Model file for the job. Use its own axes, mm. A direction names the side the tool comes from. Coordinates: 2 decimals unless noted, no trailing zeros. Order: outer loops, then holes, each group sorted by start corner. A loop starts at its lowest first (then second) coordinate and runs counter-clockwise, first axis right, second up. Notation, with made-up numbers: (30.25, 40) -> (64.25, 40) arc R16 ccw to (64.25, 67) -> close; hole circle Ø9 at (-9, 48.25). An arc over 180 degrees is marked (long way). Return JSON: item names as keys, results as strings. Group by question number.
1) Flat gauge pin, fed straight in: pin 1 (10 mm diameter, centred on x = 116.3, y = 53.8, fed in from -Z). Where does the tip first touch, or does it go through?
2) Probe line 1 (Y direction, x = 0, z = 2.1) (3 decimals); line 2 (Y direction, x = 94, z = 0.4); line 3 (X direction, y = 12, z = 2.95). List the from-to ranges inside material, lowest first.
3) Pull direction X, two halves, no side cores. Call faces 1 (the cylindrical face through (123.09, -60.69, 1.57)), 2 (the flat face through (-2, 43, 0)), 3 (the cylindrical face through (55.63, -55.73, 1.57)): +X half, -X half, draft (parallel to the pull), parting line (faces both ways), or undercut.
4) Cut at A-A (x = 15). Write the cut outline in (y, z) (3 decimals), and give its area (3 significant figures).
5) Which spindle directions (+Z, -Z, +X, -X, +Y, -Y) get a long thin tool onto all of the face, cutting with end or side? Do faces 4 (the flat face through (-2, 43, 3.175)), 5 (the cylindrical face through (-97.69, -35.29, 1.57)). Say none if no direction does.
6) Cut at C-C (z = 2.2). State how many separate pieces and enclosed holes the cut face has, and give its area (3 significant figures).
7) Cut at B-B (y = -9.5). Write the cut outline in (x, z) (3 decimals), and give its area (3 significant figures).
from build123d import *

# Parameters (mm, degrees)
F0_R     = 3.175
F1_DEPTH = 3.175


with BuildPart() as f1:
    # F0 (on Top) → F1 (new body)
    with BuildSketch(Plane.XY):
        with BuildLine():
            Line((118.650004, 62.500002), (-118.650004, 62.500002))
            ThreePointArc((-118.650004, 62.500002), (-123.140132, 60.64013), (-125.000004, 56.150002))
            Line((-125.000004, 56.150002), (-125.000004, -56.150002))
            ThreePointArc((-125.000004, -56.150002), (-123.140132, -60.64013), (-118.650004, -62.500002))
            Line((-118.650004, -62.500002), (118.650004, -62.500002))
            ThreePointArc((118.650004, -62.500002), (123.140132, -60.64013), (125.000004, -56.150002))
            Line((125.000004, -56.150002), (125.000004, 56.150002))
            ThreePointArc((125.000004, 56.150002), (123.140132, 60.64013), (118.650004, 62.500002))
        make_face()
        with Locations((-116.299996, -53.79999)):
            Circle(F0_R, mode=Mode.SUBTRACT)
        with Locations((-58.149998, -53.79999)):
            Circle(F0_R, mode=Mode.SUBTRACT)
        with Locations((-116.299996, -4e-06)):
            Circle(F0_R, mode=Mode.SUBTRACT)
        with Locations((0, -53.79999)):
            Circle(F0_R, mode=Mode.SUBTRACT)
        with Locations((58.149998, -53.79999)):
            Circle(F0_R, mode=Mode.SUBTRACT)
        with Locations((116.299996, -53.79999)):
            Circle(F0_R, mode=Mode.SUBTRACT)
        with Locations((116.299996, -4e-06)):
            Circle(F0_R, mode=Mode.SUBTRACT)
        with Locations((-116.299996, 53.79999)):
            Circle(F0_R, mode=Mode.SUBTRACT)
        with Locations((-58.149998, 53.79999)):
            Circle(F0_R, mode=Mode.SUBTRACT)
        with BuildLine():
            ThreePointArc((-99.600004, 30.750002), (-97.740132, 35.24013), (-93.250004, 37.100002))
            Line((-93.250004, 37.100002), (93.250004, 37.100002))
            ThreePointArc((93.250004, 37.100002), (97.740132, 35.24013), (99.600004, 30.750002))
            Line((99.600004, 30.750002), (99.600004, -30.750002))
            ThreePointArc((99.600004, -30.750002), (97.740132, -35.24013), (93.250004, -37.100002))
            Line((93.250004, -37.100002), (-93.250004, -37.100002))
            ThreePointArc((-93.250004, -37.100002), (-97.740132, -35.24013), (-99.600004, -30.750002))
            Line((-99.600004, -30.750002), (-99.600004, 30.750002))
        make_face(mode=Mode.SUBTRACT)
        with Locations((0, 53.79999)):
            Circle(F0_R, mode=Mode.SUBTRACT)
        with Locations((58.149998, 53.79999)):
            Circle(F0_R, mode=Mode.SUBTRACT)
        with Locations((116.299996, 53.79999)):
            Circle(F0_R, mode=Mode.SUBTRACT)
    extrude(amount=F1_DEPTH)


solid = f1.part
Answers below:
{
 "1": {"pin 1": "stops at z = 0"},
 "2": {"line 1": "y = -62.5 to -56.975, -50.625 to -37.1, 37.1 to 50.625, 56.975 to 62.5", "line 2": "y = -62.5 to -37.06, 37.06 to 62.5", "line 3": "x = -125 to -99.6, 99.6 to 125"},
 "3": {"face 1": "+X half", "face 2": "draft", "face 3": "undercut"},
 "4": {"outline": "(-62.5, 0) -> (-37.1, 0) -> (-37.1, 3.175) -> (-62.5, 3.175) -> close; (37.1, 0) -> (62.5, 0) -> (62.5, 3.175) -> (37.1, 3.175) -> close", "area": "161 mm^2"},
 "5": {"face 4": "+Z, +X, -X, +Y, -Y", "face 5": "+Z, -Z"},
 "6": {"separate pieces": "1", "enclosed holes": "13", "area": "16,100 mm^2"},
 "7": {"outline": "(-125, 0) -> (-99.6, 0) -> (-99.6, 3.175) -> (-125, 3.175) -> close; (99.6, 0) -> (125, 0) -> (125, 3.175) -> (99.6, 3.175) -> close", "area": "161 mm^2"}
}
